from build123d import *

# Parameters (mm, degrees)
F0_W      = 5
F0_H      = 142
F0_H_2    = 24
F1_DEPTH  = 100
F2_W      = 75
F2_H      = 44
F3_DEPTH  = 25
F4_W      = 34
F4_H      = 77
F5_DEPTH  = 25
F7_W      = 40
F7_H      = 77
F8_DEPTH  = 25
F9_W      = 25
F9_H      = 15
F10_DEPTH = 25


with BuildPart() as f1:
    # F0 (on Front) → F1 (new body)
    with BuildSketch(Plane.XZ):
        with Locations((-58, 0)):
            Rectangle(F0_W, F0_H)
        Polygon((-60.5, 71), (-55.5, 71), (55.5, 71), (60.5, 71), (60.5, 76), (-60.5, 76), align=None)
        Polygon((14.5, -71), (-55.5, -71), (-60.5, -71), (-60.5, -76), (9.5, -76), (14.5, -76), align=None)
        Polygon((60.5, 71), (55.5, 71), (55.5, -100), (55.5, -105), (60.5, -105), align=None)
        Polygon((55.5, -105), (55.5, -100), (14.5, -100), (9.5, -100), (9.5, -105), align=None)
        with Locations((12, -88)):
            Rectangle(F0_W, F0_H_2)
    extrude(amount=F1_DEPTH)

    # F2 (on face) → F3 (cut)
    with BuildSketch(Plane.XY.offset(76)):
        with Locations((0, -60)):
            Rectangle(F2_W, F2_H)
    extrude(amount=-F3_DEPTH, mode=Mode.SUBTRACT)

    # F4 (on face) → F5 (cut)
    with BuildSketch(Plane(origin=(0, 0, -105), x_dir=(1, 0, 0), z_dir=(0, 0, -1))):
        with Locations((33.5, 43.5)):
            Rectangle(F4_W, F4_H)
    extrude(amount=-F5_DEPTH, mode=Mode.SUBTRACT)

    # F7 (on face) → F8 (cut)
    with BuildSketch(Plane(origin=(0, 0, -76), x_dir=(1, 0, 0), z_dir=(0, 0, -1))):
        with Locations((-17.5, 43.5)):
            Rectangle(F7_W, F7_H)
    extrude(amount=-F8_DEPTH, mode=Mode.SUBTRACT)

    # F9 (on face) → F10 (cut)
    with BuildSketch(Plane.XY.offset(76)):
        with Locations((0, -22.5)):
            Rectangle(F9_W, F9_H)
    extrude(amount=-F10_DEPTH, mode=Mode.SUBTRACT)


solid = f1.part
Read the model definition and answer for the solid it produces. Units are mm, in the model's axes. A direction names the side the tool comes from. Round coordinates to 2 decimals unless told otherwise and drop trailing zeros. Loops run counter-clockwise (first coordinate to the right, second up) from the corner with the lowest first, then second, coordinate; pieces in that order, holes last. Notation, with made-up numbers: (10.5, 51) - (41.5, 51) arc R26 cw to (41.5, 86) - close; hole circle Ø4 at (13, -11.5). An arc over 180 degrees is marked (long way). One line per question, with ' | ' between items. Start each with the question number.
Q1. For a pull along Z with two mould halves and no side action, classify faces 6 (the flat face through (52, -49, -105)), 7 (the flat face through (14.5, -49, -86)), 8 (the flat face through (33, -82, -103)) as +Z half, -Z half, draft (parallel to the pull), parting line (faces both ways), or undercut.
Q2. For faces 1 (the flat face through (-37.5, -60, 74)), 2 (the flat face through (0, -30, 74)), 3 (the flat face through (14, -27, 76)), 4 (the flat face through (50.5, -43, -103)), 5 (the flat face through (-13, -27, 71)), determine the directions among +Z, -Z, +X, -X, +Y, -Y from which every point of the face is accessible in a straight line to the end or side of a thin tool.
Q3. Find the intervals of material crossed by L1, parallel to Z at x = 50, y = -87; L2, parallel to X at y = -79, z = 35.5; L3, parallel to Z at x = -2.5, y = -85, in increasing order.
Q4. Section D-D on z = -38.5 is taken. Give the vertices of the cut face in (x, y), plus the area to 3 significant figures.
Q5. Section C-C on y = -21.5 is taken. Give the vertices of the cut face in (x, z).
Q6. Flat-ended cylindrical pins translate along their axes: pin 1 (10 mm diameter, centred on x = -16.5, y = -30, fed in from -Z); pin 2 (1 mm diameter, centred on x = -9.5, y = -89, fed in from -Z). Find the tip coordinate at first contact, or state that the pin passes through.
Q7. Section B-B on x = 42 is taken. Give the vertices of the cut face in (y, z).
Q8. Section A-A on x = -41.5 is taken. Give the vertices of the cut face in (y, z), plus the area to 3 significant figures.
Established:
1) face 6: -Z half | face 7: undercut | face 8: draft
2) face 1: +Z, -Z | face 2: +Z | face 3: +Z, +X, -X, +Y, -Y | face 4: -Z | face 5: +Y, -Y
3) L1: -105 to -100, 71 to 76 | L2: -60.5 to -55.5, 55.5 to 60.5 | L3: -76 to -71, 71 to 76
4) outline: (-60.5, -100) - (-55.5, -100) - (-55.5, 0) - (-60.5, 0) - close; (55.5, -100) - (60.5, -100) - (60.5, 0) - (55.5, 0) - close | area: 1,000 mm²
5) outline: (-60.5, -76) - (-37.5, -76) - (-37.5, -71) - (-55.5, -71) - (-55.5, 71) - (-12.5, 71) - (-12.5, 76) - (-60.5, 76) - close; (2.5, -76) - (9.5, -76) - (9.5, -105) - (16.5, -105) - (16.5, -100) - (14.5, -100) - (14.5, -71) - (2.5, -71) - close; (12.5, 71) - (55.5, 71) - (55.5, -100) - (50.5, -100) - (50.5, -105) - (60.5, -105) - (60.5, 76) - (12.5, 76) - close
6) pin 1: z = 71 | pin 2: z = -76
7) outline: (-100, -105) - (-82, -105) - (-82, -100) - (-100, -100) - close; (-100, 71) - (0, 71) - (0, 76) - (-100, 76) - close; (-5, -105) - (0, -105) - (0, -100) - (-5, -100) - close
8) outline: (-100, -76) - (0, -76) - (0, -71) - (-100, -71) - close; (-100, 71) - (0, 71) - (0, 76) - (-100, 76) - close | area: 1,000 mm²
